```python
from build123d import *

# Parameters (mm, degrees)
EXTRUDE_1_DEPTH = 10
SKETCH_2_R      = 4
EXTRUDE_2_DEPTH = 15
SKETCH_3_W      = 6
SKETCH_3_H      = 6
EXTRUDE_3_DEPTH = 15


with BuildPart() as part:
    # 草图1 → 凸台-拉伸1 (new, symmetric)
    with BuildSketch(Plane.XY):
        with BuildLine():
            Line((0, 10), (40, 10))
            ThreePointArc((40, 10), (50, 0), (40, -10))
            Line((40, -10), (0, -10))
            ThreePointArc((0, -10), (-10, 0), (0, 10))
        make_face()
    extrude(amount=EXTRUDE_1_DEPTH, both=True)

    # 草图2 → 凸台-拉伸2 (add)
    with BuildSketch(Plane.XY.offset(10)):
        Circle(SKETCH_2_R)
    extrude(amount=EXTRUDE_2_DEPTH)

    # 草图3 → 凸台-拉伸3 (add)
    with BuildSketch(Plane(origin=(0, 0, -10), x_dir=(-1, 0, 0), z_dir=(0, 0, -1))):
        with Locations((-40, 0)):
            Rectangle(SKETCH_3_W, SKETCH_3_H)
    extrude(amount=EXTRUDE_3_DEPTH)


solid = part.part
```
Geometry check sheet. Reference: the model listing, model coordinates, mm. A direction names the side the tool comes from. Round coordinates to 2 decimals unless told otherwise and drop trailing zeros. Loops run counter-clockwise (first coordinate to the right, second up) from the corner with the lowest first, then second, coordinate; pieces in that order, holes last. Notation, with made-up numbers: M 39.5,76 L 43.5,76 A10 cw 43.5,82 Z; hole C -4,45 d6. An arc over 180 degrees is marked long. Return JSON: item names as keys, results as strings. Group by question number.
(1) Section check C-C, the plane z = -6.5. Enter the section's corners in (x, y), and give its area (3 significant figures).
(2) Go/stop test with flat-tipped pins: pin 1 (5 mm diameter, centred on y = -2.5, z = 3, fed in from -X); pin 2 (6.5 mm diameter, centred on y = -1, z = -14.5, fed in from +X); pin 3 (6.5 mm diameter, centred on x = 39, z = -21, fed in from -Y); pin 4 (6.5 mm diameter, centred on x = 39, z = -21, fed in from +Y). Record where each tip stops, or that it passes through.
(3) Section check A-A, the plane x = 38. Enter the section's corners in (y, z).
(4) Section check B-B, the plane y = 0. Enter the section's corners in (x, z), and give its area (3 significant figures).
(5) Set-up check for faces 1 (the face through (40, 3, -17)), 2 (the face through (40, -3, -17)), 3 (the face through (-0.867, -3.905, 17.395)): record each of +Z, -Z, +X, -X, +Y, -Y from which the full face is reachable in a straight line by a thin tool's end or side.
(6) Section check D-D, the plane x = 9.5. Enter the section's corners in (y, z), and give its area (3 significant figures).
(7) Scan lines: line 1 along Z through (x, y) = (19.5, -1.5); line 2 along X through (y, z) = (-0.5, -12); line 3 along Y through (x, z) = (-7, 0). Record each from-to range of solid material in increasing order. Write a range as [from, to].
Data:
{
 "1": {"outline": "M 0,-10 L 40,-10 A10 ccw 40,10 L 0,10 A10 ccw Z", "area": "1,110 mm²"},
 "2": {"pin 1": "x = -10", "pin 2": "x = 43", "pin 3": "y = -3", "pin 4": "y = 3"},
 "3": {"outline": "M -10,-10 L -3,-10 L -3,-25 L 3,-25 L 3,-10 L 10,-10 L 10,10 L -10,10 Z"},
 "4": {"outline": "M -10,-10 L 37,-10 L 37,-25 L 43,-25 L 43,-10 L 50,-10 L 50,10 L 4,10 L 4,25 L -4,25 L -4,10 L -10,10 Z", "area": "1,410 mm²"},
 "5": {"face 1": "-Z, +X, -X, +Y", "face 2": "-Z, +X, -X, -Y", "face 3": "+Z"},
 "6": {"outline": "M -10,-10 L 10,-10 L 10,10 L -10,10 Z", "area": "400 mm²"},
 "7": {"line 1": "[-10, 10]", "line 2": "[37, 43]", "line 3": "[-7.14, 7.14]"}
}
